```python
from build123d import *

# Parameters (mm, degrees)
SKETCH1_W           = 90
SKETCH1_H           = 20
BOSS_EXTRUDE1_DEPTH = 20
SKETCH2_W           = 90
SKETCH2_H           = 3
CUT_EXTRUDE1_DEPTH  = 10
SKETCH3_W           = 3
SKETCH3_H           = 5
CUT_EXTRUDE2_DEPTH  = 10
SKETCH4_W           = 3
SKETCH4_H           = 1.75
SKETCH4_W_2         = 2.997618753
SKETCH4_W_3         = 3.002941468
CUT_EXTRUDE3_DEPTH  = 5
SKETCH5_W           = 1.5
SKETCH5_H           = 3
BOSS_EXTRUDE2_DEPTH = 10
SKETCH6_W           = 90
SKETCH6_H           = 5
CUT_EXTRUDE4_DEPTH  = 56
SKETCH7_W           = 5
SKETCH7_H           = 5
BOSS_EXTRUDE3_DEPTH = 5
SKETCH8_R           = 1.5
CUT_EXTRUDE5_DEPTH  = 5
FILLET3_R           = 1.98


with BuildPart() as part:
    # Sketch1 → Boss-Extrude1 (new body)
    with BuildSketch(Plane.XY):
        with Locations((45, -10)):
            Rectangle(SKETCH1_W, SKETCH1_H)
    extrude(amount=BOSS_EXTRUDE1_DEPTH)

    # Sketch2 → Cut-Extrude1 (cut)
    with BuildSketch(Plane(origin=(0, 0, 0), x_dir=(1, 0, 0), z_dir=(0, 1, 0))):
        with Locations((45, -10)):
            Rectangle(SKETCH2_W, SKETCH2_H)
    extrude(amount=-CUT_EXTRUDE1_DEPTH, mode=Mode.SUBTRACT)

    # Sketch3 → Cut-Extrude2 (cut)
    with BuildSketch(Plane(origin=(0, 0, 0), x_dir=(1, 0, 0), z_dir=(0, 1, 0))):
        with Locations((11.25, -15.75)):
            Rectangle(SKETCH3_W, SKETCH3_H)
        with Locations((22.5, -15.75)):
            Rectangle(SKETCH3_W, SKETCH3_H)
        with Locations((33.75, -15.75)):
            Rectangle(SKETCH3_W, SKETCH3_H)
        with Locations((45, -15.75)):
            Rectangle(SKETCH3_W, SKETCH3_H)
        with Locations((56.25, -15.75)):
            Rectangle(SKETCH3_W, SKETCH3_H)
        with Locations((67.5, -15.75)):
            Rectangle(SKETCH3_W, SKETCH3_H)
        with Locations((78.75, -15.75)):
            Rectangle(SKETCH3_W, SKETCH3_H)
        with Locations((11.25, -4.25)):
            Rectangle(SKETCH3_W, SKETCH3_H)
        with Locations((22.5, -4.25)):
            Rectangle(SKETCH3_W, SKETCH3_H)
        with Locations((33.75, -4.25)):
            Rectangle(SKETCH3_W, SKETCH3_H)
        with Locations((45, -4.25)):
            Rectangle(SKETCH3_W, SKETCH3_H)
        with Locations((56.25, -4.25)):
            Rectangle(SKETCH3_W, SKETCH3_H)
        with Locations((67.5, -4.25)):
            Rectangle(SKETCH3_W, SKETCH3_H)
        with Locations((78.75, -4.25)):
            Rectangle(SKETCH3_W, SKETCH3_H)
    extrude(amount=-CUT_EXTRUDE2_DEPTH, mode=Mode.SUBTRACT)

    # Sketch4 → Cut-Extrude3 (cut)
    with BuildSketch(Plane(origin=(0, 0, 0), x_dir=(1, 0, 0), z_dir=(0, 1, 0))):
        with Locations((56.25, -19.125)):
            Rectangle(SKETCH4_W, SKETCH4_H)
        with Locations((67.5, -19.125)):
            Rectangle(SKETCH4_W, SKETCH4_H)
        Polygon((77.25, -18.25), (77.25, -20), (80.252941468, -20), (80.252941468, -18.25), (80.25, -18.25), align=None)
        with Locations((45, -19.125)):
            Rectangle(SKETCH4_W, SKETCH4_H)
        with Locations((33.748809377, -19.125)):
            Rectangle(SKETCH4_W_2, SKETCH4_H)
        with Locations((22.5, -19.125)):
            Rectangle(SKETCH4_W, SKETCH4_H)
        with Locations((11.25, -19.125)):
            Rectangle(SKETCH4_W, SKETCH4_H)
        with Locations((22.5, -0.875)):
            Rectangle(SKETCH4_W, SKETCH4_H)
        with Locations((33.748809377, -0.875)):
            Rectangle(SKETCH4_W_2, SKETCH4_H)
        with Locations((45, -0.875)):
            Rectangle(SKETCH4_W, SKETCH4_H)
        with Locations((56.25, -0.875)):
            Rectangle(SKETCH4_W, SKETCH4_H)
        with Locations((67.5, -0.875)):
            Rectangle(SKETCH4_W, SKETCH4_H)
        with Locations((78.751470734, -0.875)):
            Rectangle(SKETCH4_W_3, SKETCH4_H)
        with Locations((11.25, -0.875)):
            Rectangle(SKETCH4_W, SKETCH4_H)
    extrude(amount=-CUT_EXTRUDE3_DEPTH, mode=Mode.SUBTRACT)

    # Sketch5 → Boss-Extrude2 (add)
    with BuildSketch(Plane(origin=(0, -10, 0), x_dir=(1, 0, 0), z_dir=(0, 1, 0))):
        with Locations((0.75, -10)):
            Rectangle(SKETCH5_W, SKETCH5_H)
        with Locations((89.25, -10)):
            Rectangle(SKETCH5_W, SKETCH5_H)
    extrude(amount=BOSS_EXTRUDE2_DEPTH)

    # Sketch6 → Cut-Extrude4 (cut)
    with BuildSketch(Plane.XY.offset(20)):
        with Locations((45, -17.5)):
            Rectangle(SKETCH6_W, SKETCH6_H)
    extrude(amount=-CUT_EXTRUDE4_DEPTH, mode=Mode.SUBTRACT)

    # Sketch7 → Boss-Extrude3 (add)
    with BuildSketch(Plane.XZ.offset(15)):
        with Locations((2.5, 22.5)):
            Rectangle(SKETCH7_W, SKETCH7_H)
        with Locations((2.5, -2.5)):
            Rectangle(SKETCH7_W, SKETCH7_H)
    extrude(amount=-BOSS_EXTRUDE3_DEPTH)

    # Sketch8 → Cut-Extrude5 (cut)
    with BuildSketch(Plane(origin=(0, -10, 0), x_dir=(1, 0, 0), z_dir=(0, 1, 0))):
        with Locations((2.5, 2.5)):
            Circle(SKETCH8_R)
        with Locations((2.5, -22.5)):
            Circle(SKETCH8_R)
    extrude(amount=-CUT_EXTRUDE5_DEPTH, mode=Mode.SUBTRACT)

    # Fillet3
    fillet3_edges = [part.edges().sort_by_distance(p)[0] for p in [
        (0, -12.5, 25),
        (5, -12.5, 25),
        (0, -12.5, -5),
        (5, -12.5, -5),
    ]]
    fillet(fillet3_edges, radius=FILLET3_R)


solid = part.part
```
The listing builds one solid part. Answer for the finished solid, in the listing's coordinates (mm). A direction names the side the tool comes from. Give positions to 0.01 mm unless a question says otherwise; leave off trailing zeros. Order: outer loops, then holes, each group sorted by start corner. A loop starts at its lowest first (then second) coordinate and runs counter-clockwise, first axis right, second up. Notation, with made-up numbers: M -2.75,-26.5 L 51.25,-26.5 A14 ccw 51.25,-5.5 Z; hole C 74.5,19 d7. An arc over 180 degrees is marked long. Put each result on its own line as item: value. Start each with the question number.
Item 1: Flat-ended cylindrical pins translate along their axes: P1, Ø1.5, axis at x = 55.5, y = -6.5, coming from the +Z side; P2, Ø5.5, axis at y = -6.5, z = 4, coming from the -X side; P3, Ø2.5, axis at x = 67, y = -8.5, coming from the -Z side. Find the tip coordinate at first contact, or state that the pin passes through.
Item 2: Find the intervals of material crossed by line 1 along Z through (x, y) = (2.5, -12.1); line 2 along Z through (x, y) = (15, -2.75); line 3 along Z through (x, y) = (12.5, -2.5), in increasing order.
Item 3: Which of the six approach directions +Z, -Z, +X, -X, +Y, -Y give full straight-line access (tool end or side, diameter ignored) to faces 5 (the face through (67, -10, 16)), 6 (the face through (1, -10, -1)), 7 (the face through (80.253, -2, 1)), 8 (the face through (1, -10, 21))?
Item 4: The part is cut by section B-B, the plane x = 44.5. Determine the outline of the cut face in (y, z).
Item 5: The part is cut by section C-C, the plane z = 9.5. Determine the outline of the cut face in (x, y), and give its area (3 significant figures).
Item 6: For a pull along Z with two mould halves and no side action, classify faces 1 (the face through (35.248, -2, 19)), 2 (the face through (77.25, -5, 3)), 3 (the face through (44, -10, 10)), 4 (the face through (4.4, -12.46, -4.44)) as +Z half, -Z half, draft (parallel to the pull), parting line (faces both ways), or undercut.
Item 7: The part is cut by section A-A, the plane y = -13. Determine the outline of the cut face in (x, z).
Answer key:
1. P1: stops at z = 20
1. P2: stops at x = 0
1. P3: stops at z = 0
2. line 1: z = -5 to -4, -1 to 21, 24 to 25
2. line 2: z = 0 to 8.5, 11.5 to 20
2. line 3: z = 6.75 to 8.5, 11.5 to 13.25
3. face 5: +Y
3. face 6: -Z, +X, -X, +Y
3. face 7: -Z, +Y
3. face 8: +Z, +X, -X, +Y
4. outline: M -15,0 L -5,0 L -5,1.75 L -10,1.75 L -10,6.75 L 0,6.75 L 0,8.5 L -10,8.5 L -10,11.5 L 0,11.5 L 0,13.25 L -10,13.25 L -10,18.25 L -5,18.25 L -5,20 L -15,20 Z
5. outline: M 0,-15 L 90,-15 L 90,0 L 88.5,0 L 88.5,-10 L 1.5,-10 L 1.5,0 L 0,0 Z
5. area: 480 mm²
6. face 1: draft
6. face 2: undercut
6. face 3: undercut
6. face 4: -Z half
7. outline: M 0,-3.02 A1.98 ccw 1.98,-5 L 3.02,-5 A1.98 ccw 5,-3.02 L 5,0 L 90,0 L 90,20 L 5,20 L 5,23.02 A1.98 ccw 3.02,25 L 1.98,25 A1.98 ccw 0,23.02 Z; hole C 2.5,-2.5 d3; hole C 2.5,22.5 d3
